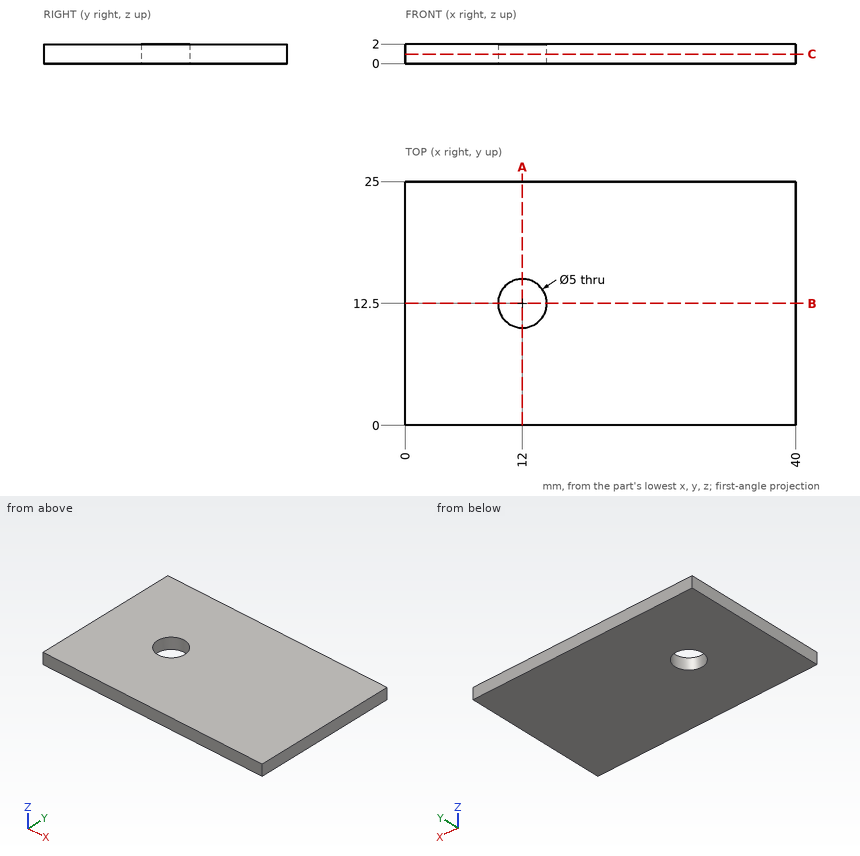
Geometry: see drawing. Coordinates: mm, zero at the bounding-box minimum. Round coordinates to 2 decimals unless told otherwise and drop trailing zeros. Loops run counter-clockwise (first coordinate to the right, second up) from the corner with the lowest first, then second, coordinate; pieces in that order, holes last. Notation, with made-up numbers: (66.25, 46) -> (71.25, 46) arc R10 ccw to (71.25, 58) -> close; hole circle Ø2 at (38.5, 43.25). An arc over 180 degrees is marked (long way). Use one line per item in the form item = value. Start each with the question number.
Item 1: Section query C-C on z = 0.95. Return the cut outline in (x, y), then the cut area to 3 significant figures.
Item 2: Section query B-B on y = 12.5. Return the cut outline in (x, z), then the cut area to 3 significant figures.
Item 3: Material intervals for L1, parallel to Y at x = 13.5, z = 0.5; L2, parallel to Y at x = 11, z = 1.4; L3, parallel to X at y = 13, z = 0.65, sorted ascending. Write a range as from..to.
Item 4: Contact query for a flat-ended pin moving along its axis: pin 1 Ø3 at (x, y) = (12, 12.5) entering from -Z. Output: stop coordinate, or through.
Item 5: Section query A-A on x = 12. Return the cut outline in (y, z), then the cut area to 3 significant figures.
Ans:
q1.outline = (0, 0) -> (40, 0) -> (40, 25) -> (0, 25) -> close; hole circle Ø5 at (12, 12.5)
q1.area = 980 mm^2
q2.outline = (0, 0) -> (9.5, 0) -> (9.5, 2) -> (0, 2) -> close; (14.5, 0) -> (40, 0) -> (40, 2) -> (14.5, 2) -> close
q2.area = 70.0 mm^2
q3.L1 = 0..10.5, 14.5..25
q3.L2 = 0..10.21, 14.79..25
q3.L3 = 0..9.55, 14.45..40
q4.pin_1 = through
q5.outline = (0, 0) -> (10, 0) -> (10, 2) -> (0, 2) -> close; (15, 0) -> (25, 0) -> (25, 2) -> (15, 2) -> close
q5.area = 40.0 mm^2
